Geometry check sheet. Reference: drawing and pictorial views, mm from the part's lowest x, y, z. Round coordinates to 2 decimals unless told otherwise and drop trailing zeros. Write each loop counter-clockwise with the first axis right and the second up, starting at its lowest first coordinate (ties: lowest second). Pieces come first, ordered by that corner, then holes. Notation, with made-up numbers: M 36,55.5 L 67,55.5 A11 cw 67,68.5 Z; hole C 78,27.25 d11. An arc over 180 degrees is marked long. One line per item, written item: value. Start each with the question number.
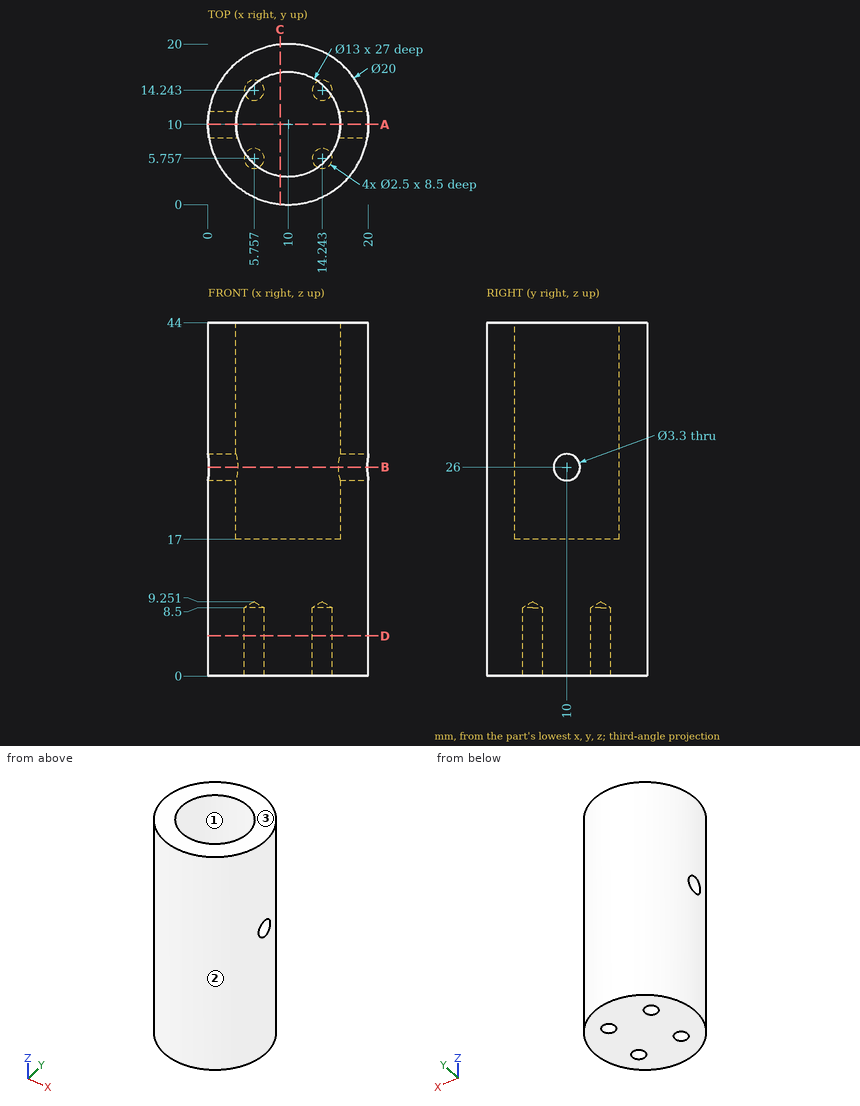
1) Cross-section at D-D (z = 5). Record the boundary of the cut face in (x, y).
2) Thickness scan on line 1 (Z direction, x = 10.5, y = 10.5); line 2 (X direction, y = 15.25, z = 37.5) (1 decimal); line 3 (Y direction, x = 14.75, z = 28) (1 decimal). Record the ranges inside material, lowest first.
3) Cross-section at A-A (y = 10). Record the boundary of the cut face in (x, z).
4) Cross-section at C-C (x = 9). Record the boundary of the cut face in (y, z).
5) Cross-section at B-B (z = 26). Record the boundary of the cut face in (x, y).
6) Gauge pin test, flat ends, axial feed: pin 1 Ø4 at (x, z) = (5, 13.5) entering from -Y; pin 2 Ø3 at (y, z) = (10, 26) entering from -X; pin 3 Ø5 at (x, z) = (2.5, 10) entering from +Y; pin 4 Ø4 at (x, y) = (9, 13) entering from +Z. Record the tip position at first contact, or that the pin passes through.
7) Mould release check, pull along X, two halves, no side actions. Record for the marked faces 1, 2 and 3: pulls with the +X half, pulls with the -X half, needs draft (parallel to the pull), parting line crosses it, or undercut.
Results below:
1. outline: C 10,10 d20; hole C 5.76,5.76 d2.5; hole C 5.76,14.24 d2.5; hole C 14.24,5.76 d2.5; hole C 14.24,14.24 d2.5
2. line 1: z = 0 to 17
2. line 2: x = 1.5 to 6.2, 13.8 to 18.5
2. line 3: y = 1.2 to 5.6, 14.4 to 18.8
3. outline: M 0,0 L 20,0 L 20,24.35 L 16.5,24.35 L 16.5,17 L 3.5,17 L 3.5,24.35 L 0,24.35 Z; M 0,27.65 L 3.5,27.65 L 3.5,44 L 0,44 Z; M 16.5,27.65 L 20,27.65 L 20,44 L 16.5,44 Z
4. outline: M 0.05,0 L 19.95,0 L 19.95,44 L 16.42,44 L 16.42,17 L 3.58,17 L 3.58,44 L 0.05,44 Z
5. outline: M 0.14,8.35 A10 ccw 19.86,8.35 L 16.29,8.35 A6.5 cw 3.71,8.35 Z; M 0.14,11.65 L 3.71,11.65 A6.5 cw 16.29,11.65 L 19.86,11.65 A10 ccw Z
6. pin 1: stops at y = 0.46
6. pin 2: passes through
6. pin 3: stops at y = 18.66
6. pin 4: stops at z = 17
7. face 1: undercut
7. face 2: parting line crosses it
7. face 3: needs draft
